from build123d import *

# Parameters (mm, degrees)
SKETCH_1_R          = 17.5
EXTRUDE_1_DEPTH     = 5
SKETCH_2_R          = 1.5
SKETCH_2_R_2        = 4
CUT_EXTRUDE_1_DEPTH = 5


with BuildPart() as part:
    # 草图1 → 凸台-拉伸1 (new body)
    with BuildSketch(Plane.XY):
        Circle(SKETCH_1_R)
    extrude(amount=EXTRUDE_1_DEPTH)

    # 草图2 → 切除-拉伸1 (cut)
    with BuildSketch(Plane.XY.offset(5)):
        with Locations((0, 13.5)):
            Circle(SKETCH_2_R)
        with Locations((11.691342951, 6.75)):
            Circle(SKETCH_2_R)
        with Locations((11.691342951, -6.75)):
            Circle(SKETCH_2_R)
        Circle(SKETCH_2_R_2)
        with Locations((0, -13.5)):
            Circle(SKETCH_2_R)
        with Locations((-11.691342951, -6.75)):
            Circle(SKETCH_2_R)
        with Locations((-11.691342951, 6.75)):
            Circle(SKETCH_2_R)
    extrude(amount=-CUT_EXTRUDE_1_DEPTH, mode=Mode.SUBTRACT)


solid = part.part
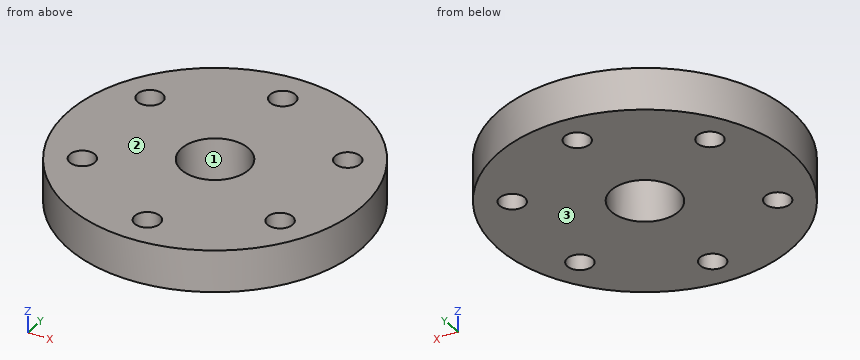
Can you work these out from the model? Positions are in its coordinate system, mm. Face numbers are marked on the shaded views. Give positions to 0.01 mm unless a question says otherwise; leave off trailing zeros. Loops run counter-clockwise (first coordinate to the right, second up) from the corner with the lowest first, then second, coordinate; pieces in that order, holes last. Notation, with made-up numbers: (34, 47) - (89, 47) arc R8 ccw to (89, 56) - close; hole circle Ø10 at (83, -1). An arc over 180 degrees is marked (long way). Return JSON: item names as keys, results as strings.
1. I want a section at C-C on z = 1.05. Please give me the cut outline in (x, y).
Output values:
{"outline": "circle Ø35 at (0, 0); hole circle Ø3 at (-11.69, -6.75); hole circle Ø3 at (-11.69, 6.75); hole circle Ø8 at (0, 0); hole circle Ø3 at (0, -13.5); hole circle Ø3 at (0, 13.5); hole circle Ø3 at (11.69, -6.75); hole circle Ø3 at (11.69, 6.75)"}
2. I want a section at B-B on y = 0. Please give me the cut outline in (x, z), and give its area (3 significant figures).
Output values:
{"outline": "(-17.5, 0) - (-4, 0) - (-4, 5) - (-17.5, 5) - close; (4, 0) - (17.5, 0) - (17.5, 5) - (4, 5) - close", "area": "135 mm²"}
3. I want a section at A-A on x = 0. Please give me the cut outline in (y, z).
Output values:
{"outline": "(-17.5, 0) - (-15, 0) - (-15, 5) - (-17.5, 5) - close; (-12, 0) - (-4, 0) - (-4, 5) - (-12, 5) - close; (4, 0) - (12, 0) - (12, 5) - (4, 5) - close; (15, 0) - (17.5, 0) - (17.5, 5) - (15, 5) - close"}
4. I want a section at D-D on y = -6.75. Please give me the cut outline in (x, z).
Output values:
{"outline": "(-16.15, 0) - (-13.19, 0) - (-13.19, 5) - (-16.15, 5) - close; (-10.19, 0) - (10.19, 0) - (10.19, 5) - (-10.19, 5) - close; (13.19, 0) - (16.15, 0) - (16.15, 5) - (13.19, 5) - close"}
5. We'd pull the mould along Z, two halves only. Please class the marked faces 1, 2 and 3: +Z half, -Z half, draft (parallel to the pull), parting line (faces both ways), or undercut.
Output values:
{"face 1": "draft", "face 2": "+Z half", "face 3": "-Z half"}
6. If I drill on line 1 (Y direction, x = -11, z = 2.4); line 2 (Y direction, x = 0.5, z = 0.95); line 3 (Y direction, x = 0, z = 4.6), over which ranges is the centre line in solid material (lowest first)?
Output values:
{"line 1": "y = -13.61 to -8.08, -5.42 to 5.42, 8.08 to 13.61", "line 2": "y = -17.49 to -14.91, -12.09 to -3.97, 3.97 to 12.09, 14.91 to 17.49", "line 3": "y = -17.5 to -15, -12 to -4, 4 to 12, 15 to 17.5"}
7. I'm going to push flat-ended pins straight in: pin 1 Ø1 at (y, z) = (7, 4) entering from -X; pin 2 Ø1.5 at (x, z) = (-4, 3) entering from -Y. Where does each tip first touch, or does it pass through?
Output values:
{"pin 1": "stops at x = -16.25", "pin 2": "stops at y = -17.2"}
